Verification items for the finished model (mm, model axes). Face numbers are marked on the shaded views. A direction names the side the tool comes from. Give positions to 0.01 mm unless a question says otherwise; leave off trailing zeros. Order: outer loops, then holes, each group sorted by start corner. A loop starts at its lowest first (then second) coordinate and runs counter-clockwise, first axis right, second up. Notation, with made-up numbers: (13, -9.75) - (57, -9.75) arc R23 ccw to (57, 6.25) - close; hole circle Ø10 at (40.25, 4). An arc over 180 degrees is marked (long way). Answer as a JSON object with one key per item and string values.
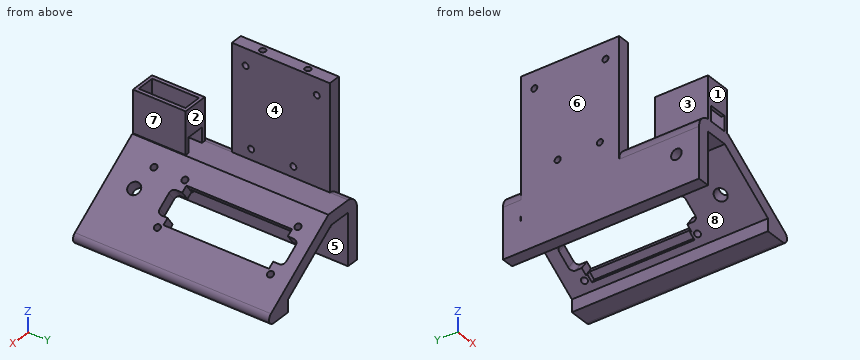
```python
from build123d import *

# Parameters (mm, degrees)
F1_DEPTH       = 80
F1_DEPTH_BACK  = 50
F2_R           = 2
F3_DEPTH       = 25
F4_W           = 17
F4_H           = 35
F4_W_2         = 12
F4_H_2         = 31
F5_DEPTH       = 28
F6_W           = 6
F6_H           = 10
F7_DEPTH       = 35.001
F8_R           = 4
F8_R_2         = 2
F9_DEPTH       = 25
F10_R          = 3.5
F11_DEPTH      = 8
F12_W          = 8
F12_H          = 65
F13_DEPTH      = 70
F13_DEPTH_BACK = 25
F14_R          = 2
F15_DEPTH      = 25
F16_R          = 2
F17_DEPTH      = 25
F18_W          = 35
F18_H          = 68
F19_DEPTH      = 3.5


with BuildPart() as f1:
    # F0 (on Front) → F1 (new body, two sides)
    with BuildSketch(Plane.XZ) as f1_sk:
        with BuildLine():
            Line((7.5, 34.4145861811), (45.9434284027, 7.4962078188))
            Line((45.9434284027, 7.4962078188), (45.9434284027, -0.7233918228))
            Line((45.9434284027, -0.7233918228), (58.9434284027, -0.7233918228))
            ThreePointArc((58.9434284027, -0.7233918228), (62.7582962057, 2.0737849791), (61.2377341481, 6.5532163543))
            Line((61.2377341481, 6.5532163543), (10.022390311, 42.4145861811))
            Line((10.022390311, 42.4145861811), (-7.5, 42.4145861811))
            ThreePointArc((-7.5, 42.4145861811), (-13.2082039325, 39.4703142711), (-15.5, 33.4703142711))
            Line((-15.5, 33.4703142711), (-15.5, 0))
            Line((-15.5, 0), (-7.5, 0))
            Line((-7.5, 0), (-7.5, 34.4145861811))
            Line((-7.5, 34.4145861811), (7.5, 34.4145861811))
        make_face()
    extrude(amount=F1_DEPTH)
    extrude(f1_sk.sketch, amount=-F1_DEPTH_BACK)

    # F2 (on face) → F3 (cut)
    with BuildSketch(Plane(origin=(23.2256022942, 0, 33.1695976219), x_dir=(0.8191520443, 0, -0.5735764364), z_dir=(0.5735764364, 0, 0.8191520443))):
        with BuildLine():
            Line((-1.0957553681, 35), (-1.0957553681, -35))
            Line((-1.0957553681, -35), (3.4042446319, -35))
            Line((3.4042446319, -35), (3.4042446319, -39))
            ThreePointArc((3.4042446319, -39), (4.2829242884, -41.1213203436), (6.4042446319, -42))
            Line((6.4042446319, -42), (16.4042446319, -42))
            ThreePointArc((16.4042446319, -42), (18.5255649755, -41.1213203436), (19.4042446319, -39))
            Line((19.4042446319, -39), (19.4042446319, -35))
            Line((19.4042446319, -35), (23.9042446319, -35))
            Line((23.9042446319, -35), (23.9042446319, 35))
            Line((23.9042446319, 35), (19.4042446319, 35))
            Line((19.4042446319, 35), (3.4042446319, 35))
            Line((3.4042446319, 35), (-1.0957553681, 35))
        make_face()
        with BuildLine():
            Line((3.4042446319, 35.0351855159), (3.4042446319, 35))
            Line((3.4042446319, 35), (19.4042446319, 35))
            Line((19.4042446319, 35), (19.4042446319, 39))
            ThreePointArc((19.4042446319, 39), (18.5255649755, 41.1213203436), (16.4042446319, 42))
            Line((16.4042446319, 42), (6.4042446319, 42))
            ThreePointArc((6.4042446319, 42), (4.2829242884, 41.1213203436), (3.4042446319, 39))
            Line((3.4042446319, 39), (3.4042446319, 35.0351855159))
        make_face()
        with Locations((-3.5957553681, -37.5)):
            Circle(F2_R)
        with Locations((-3.5957553681, 37.5)):
            Circle(F2_R)
        with Locations((26.4042446319, 37.5)):
            Circle(F2_R)
        with Locations((26.4042446319, -37.5)):
            Circle(F2_R)
    extrude(amount=-F3_DEPTH, mode=Mode.SUBTRACT)

    # F4 (on face) → F5 (join)
    with BuildSketch(Plane.XY.offset(42.4145861811)):
        with Locations((1, -62.5)):
            Rectangle(F4_W, F4_H)
        with Locations((1, -62.5)):
            Rectangle(F4_W_2, F4_H_2, mode=Mode.SUBTRACT)
    extrude(amount=F5_DEPTH)

    # F6 (on face) → F7 (cut, through all)
    with BuildSketch(Plane(origin=(0, -45, 0), x_dir=(-1, 0, 0), z_dir=(0, 1, 0))):
        with Locations((-4, 47.4145861811)):
            Rectangle(F6_W, F6_H)
        with Locations((2, 47.4145861811)):
            Rectangle(F6_W, F6_H)
    extrude(amount=-F7_DEPTH, mode=Mode.SUBTRACT)

    # F8 (on face) → F9 (cut)
    with BuildSketch(Plane(origin=(23.2256022942, 0, 33.1695976219), x_dir=(0.8191520443, 0, -0.5735764364), z_dir=(0.5735764364, 0, 0.8191520443))):
        with Locations((11.4042446319, -62)):
            Circle(F8_R)
        with Locations((-3.5957553681, -58)):
            Circle(F8_R_2)
    extrude(amount=-F9_DEPTH, mode=Mode.SUBTRACT)

    # F10 (on face) → F11 (cut, through all)
    with BuildSketch(Plane(origin=(-15.5, 0, 0), x_dir=(0, -1, 0), z_dir=(-1, 0, 0))):
        with Locations((-35, 21.4703142711)):
            Circle(F10_R)
        with Locations((65, 21.4703142711)):
            Circle(F10_R)
    extrude(amount=-F11_DEPTH, mode=Mode.SUBTRACT)

    # F12 (on face) → F13 (join, two sides)
    with BuildSketch(Plane.XY.offset(42.4145861811)) as f13_sk:
        with Locations((-11.5, 5.4507081211)):
            Rectangle(F12_W, F12_H)
    extrude(amount=F13_DEPTH)
    extrude(f13_sk.sketch, amount=-F13_DEPTH_BACK)

    # F14 (on face) → F15 (cut)
    with BuildSketch(Plane.XY.offset(112.4145861811)):
        with Locations((-11.5, -9.5492918789)):
            Circle(F14_R)
        with Locations((-11.5, 20.4507081211)):
            Circle(F14_R)
    extrude(amount=-F15_DEPTH, mode=Mode.SUBTRACT)

    # F16 (on face) → F17 (cut)
    with BuildSketch(Plane.YZ.offset(-7.5)):
        with Locations((13.7650537365, 49.4145861811)):
            Circle(F16_R)
        with Locations((-14.2349462635, 49.4145861811)):
            Circle(F16_R)
        with Locations((29.2650537365, 101.3145861811)):
            Circle(F16_R)
        with Locations((-17.9349462635, 101.3145861811)):
            Circle(F16_R)
    extrude(amount=-F17_DEPTH, mode=Mode.SUBTRACT)

    # F18 (on face) → F19 (cut)
    with BuildSketch(Plane(origin=(18.6369908034, 0, 26.6163812675), x_dir=(0.8191520443, 0, -0.5735764364), z_dir=(-0.5735764364, 0, -0.8191520443))):
        with Locations((11.4042446319, 0)):
            Rectangle(F18_W, F18_H)
    extrude(amount=-F19_DEPTH, mode=Mode.SUBTRACT)


solid = f1.part
```
(1) Section check D-D (x = 50). Record the cut outline in (y, z).
Computed values:
{"outline": "(-80, -0.72) - (50, -0.72) - (50, 14.42) - (-80, 14.42) - close"}
(2) Material ranges on line 1 along Y through (x, z) = (-11.5, 104.5); line 2 along Y through (x, z) = (40, 19); line 3 along X through (y, z) = (24.5, 32.5), recorded low to high. Write a range as [from, to].
Computed values:
{"line 1": "y = [-27.05, -11.55], [-7.55, 18.45], [22.45, 37.95]", "line 2": "y = [-80, -35], [35, 50]", "line 3": "x = [-15.5, -7.5], [10.23, 15.32], [16.34, 21.42]"}
(3) Section check B-B (x = -11.5). Record the cut outline in (y, z).
Computed values:
{"outline": "(-80, 0) - (50, 0) - (50, 40.95) - (37.95, 40.95) - (37.95, 112.41) - (22.45, 112.41) - (22.45, 87.41) - (18.45, 87.41) - (18.45, 112.41) - (-7.55, 112.41) - (-7.55, 87.41) - (-11.55, 87.41) - (-11.55, 112.41) - (-27.05, 112.41) - (-27.05, 40.95) - (-80, 40.95) - close; hole circle Ø7 at (-65, 21.47); hole circle Ø4 at (-17.93, 101.31); hole circle Ø4 at (-14.23, 49.41); hole circle Ø4 at (13.77, 49.41); hole circle Ø4 at (29.27, 101.31); hole (37.95, 19.59) arc R3.5 ccw to (37.95, 23.35) - close"}
(4) Section check C-C (z = 94). Record the cut outline in (x, y).
Computed values:
{"outline": "(-15.5, -27.05) - (-7.5, -27.05) - (-7.5, 37.95) - (-15.5, 37.95) - close; hole circle Ø4 at (-11.5, -9.55); hole circle Ø4 at (-11.5, 20.45)"}
(5) Section check A-A (z = 45). Record the cut outline in (x, y), then the cut area to 3 significant figures.
Computed values:
{"outline": "(-15.5, -27.05) - (-7.5, -27.05) - (-7.5, 37.95) - (-15.5, 37.95) - close; (-7.5, -80) - (-5, -80) - (-5, -45) - (-7.5, -45) - close; (7, -80) - (9.5, -80) - (9.5, -45) - (7, -45) - close", "area": "695 mm²"}
(6) Access from +Z, -Z, +X, -X, +Y, -Y to the whole of each face (thin tool, end or side, straight path). Record for the marked faces 1, 2, 3 and 4.
Computed values:
{"face 1": "+Z, -Z, +X, -X, -Y", "face 2": "+Z, +X, -X, +Y", "face 3": "+Z, -X, -Y", "face 4": "+Z, +X, +Y"}
(7) Gauge pin test, flat ends, axial feed: pin 1 Ø4.5 at (y, z) = (13.77, 49.41) entering from +X; pin 2 Ø5 at (x, y) = (46, -1.5) entering from +Z; pin 3 Ø6.5 at (x, z) = (-12, 62.5) entering from -Y. Record the tip position at first contact, or that the pin passes through.
Computed values:
{"pin 1": "stops at x = -7.5", "pin 2": "stops at z = 18.97", "pin 3": "stops at y = -27.05"}
(8) Release check for a two-part mould opening along X. For the marked faces 5, 6, 7 and 8 record: pulls with the +X half, pulls with the -X half, needs draft (parallel to the pull), parting line crosses it, or undercut.
Computed values:
{"face 5": "undercut", "face 6": "pulls with the -X half", "face 7": "pulls with the +X half", "face 8": "undercut"}
